Geometry check sheet. Reference: drawing and pictorial views, mm from the part's lowest x, y, z. A direction names the side the tool comes from. Coordinates: 2 decimals unless noted, no trailing zeros. Loops run counter-clockwise (first coordinate to the right, second up) from the corner with the lowest first, then second, coordinate; pieces in that order, holes last.
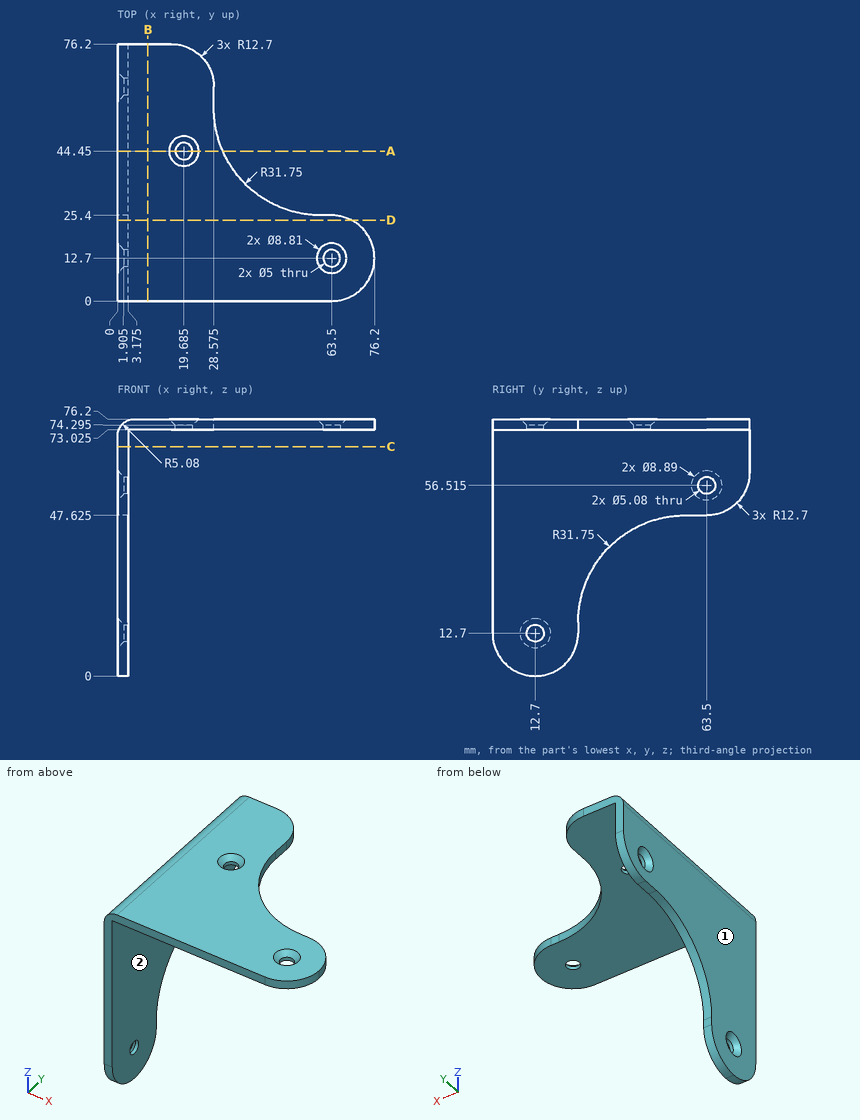
1) Section check D-D on y = 24. Record the cut outline in (x, z) (1 decimal).
Data:
outline: (0, 6.9) - (3.2, 6.9) - (3.2, 73) - (69.3, 73) - (69.3, 76.2) - (5.1, 76.2) arc R5.1 ccw to (0, 71.1) - close
2) Section check B-B on x = 9. Record the cut outline in (y, z) (3 decimals).
Data:
outline: (0, 73.025) - (76.2, 73.025) - (76.2, 76.2) - (0, 76.2) - close
3) Depth check by flat-ended pin: pin 1 (1 mm diameter, centred on x = 1, z = 15, fed in from +Y); pin 2 (22 mm diameter, centred on y = 22, z = 37, fed in from +X) (3 decimals); pin 3 (4 mm diameter, centred on x = 31.5, y = 13, fed in from -Z) (3 decimals). Enter the tip coordinate at first touch or a pass-through.
Data:
pin 1: stops at y = 25.4
pin 2: stops at x = 3.175
pin 3: stops at z = 73.025
4) Section check A-A on y = 44.45. Record the cut outline in (x, z) (1 decimal).
Data:
outline: (0, 45) - (3.2, 45) - (3.2, 73) - (17.2, 73) - (17.2, 74.3) - (15.3, 76.2) - (5.1, 76.2) arc R5.1 ccw to (0, 71.1) - close; (22.2, 73) - (31.2, 73) - (31.2, 76.2) - (24.1, 76.2) - (22.2, 74.3) - close
5) Material ranges on probe 1 along Y at (x, z) = (63.5, 73.7); probe 2 along X at (y, z) = (65, 64) (3 decimals); probe 3 along Z at (x, y) = (35, 11) (3 decimals), recorded low to high.
Data:
probe 1: y = 0 to 10.2, 15.2 to 25.4
probe 2: x = 0 to 3.175
probe 3: z = 73.025 to 76.2
6) Access from +Z, -Z, +X, -X, +Y, -Y to the whole of each face (thin tool, end or side, straight path). Record for the marked faces 1 and 2.
Data:
face 1: +Z, -Z, -X, +Y, -Y
face 2: -Z, +X, +Y, -Y
7) Section check C-C on z = 68. Record the cut outline in (x, y) (3 decimals), and give its area (3 significant figures).
Data:
outline: (0, 0) - (3.175, 0) - (3.175, 76.2) - (0, 76.2) - close
area: 242 mm2
